Geometry: final body of the model. Coordinates: model frame, mm. Face numbers are marked on the shaded views. A direction names the side the tool comes from. Coordinates: 2 decimals unless noted, no trailing zeros. Loops run counter-clockwise (first coordinate to the right, second up) from the corner with the lowest first, then second, coordinate; pieces in that order, holes last. Notation, with made-up numbers: (61.25, 41.5) -> (80.25, 41.5) arc R19 cw to (80.25, 46.5) -> close; hole circle Ø10 at (7, -14). An arc over 180 degrees is marked (long way). One line per item, written item: value. Start each with the question number.
Item 1: Section query B-B on y = -4.5. Return loops of the section in (x, z).
Item 2: Mould query, pull axis Z, two halves, no side actions, for the marked faces 3, 4 and 5. Classes: +Z half, -Z half, draft (parallel to the pull), parting line (faces both ways), or undercut.
Item 3: Contact query for flat-ended pins moving along their axis: pin 1 Ø1.5 at (x, z) = (20, -10) entering from -Y; pin 2 Ø7.5 at (y, z) = (-12.7, 0) entering from -X; pin 3 Ø1 at (x, y) = (26.5, -13) entering from -Z. Output: stop coordinate, or through.
Item 4: Section query D-D on y = -12.7. Give the number of separate pieces and of enclosed holes in the cut face, then the cut area to 3 significant figures.
Item 5: Set-up query: the marked faces 1 and 2. Return all of +Z, -Z, +X, -X, +Y, -Y with unobstructed straight access to the full face (end or side cutting, diameter ignored); none if empty.
Item 6: Ray query, probe 1 along X at (y, z) = (-10.5, 7); probe 2 along Y at (x, z) = (0, 49) (3 decimals). Return the intervals inside material, ascending. Write a range as from..to.
Item 7: Section query C-C on z = 0. Return loops of the section in (x, y).
Item 8: Section query A-A on x = 0. Return loops of the section in (y, z) (3 decimals), then the cut area to 3 significant figures.
from build123d import *

# Parameters (mm, degrees)
F1_DEPTH = 25.4
F2_T     = -2.54
F4_D     = 6.35
F6_D     = 12.7


with BuildPart() as f1:
    # F0 (on Front) → F1 (new body)
    with BuildSketch(Plane.XZ):
        Polygon((50.8, -21.042049), (50.8, 21.042049), (21.042049, 50.8), (-21.042049, 50.8), (-21.042049, -50.8), (0, -50.8), (21.042049, -50.8), align=None)
        Polygon((-21.042049, -50.8), (-21.042049, 50.8), (-50.8, 21.042049), (-50.8, -21.042049), align=None)
    extrude(amount=F1_DEPTH)

    # F2
    f2_openings = [f1.faces().sort_by_distance(p)[0] for p in [
        (0, -25.4, 0),
    ]]
    offset(amount=F2_T, openings=f2_openings)

    # F4 (through all)
    with Locations(Plane(origin=(0, 0, -50.8), x_dir=(1, 0, 0), z_dir=(0, 0, -1))):
        with Locations((0, 12.7)):
            Hole(F4_D / 2)

    # F6 (through all)
    with Locations(Plane.YZ.offset(50.8)):
        with Locations((-12.7, 0)):
            Hole(F6_D / 2)


solid = f1.part
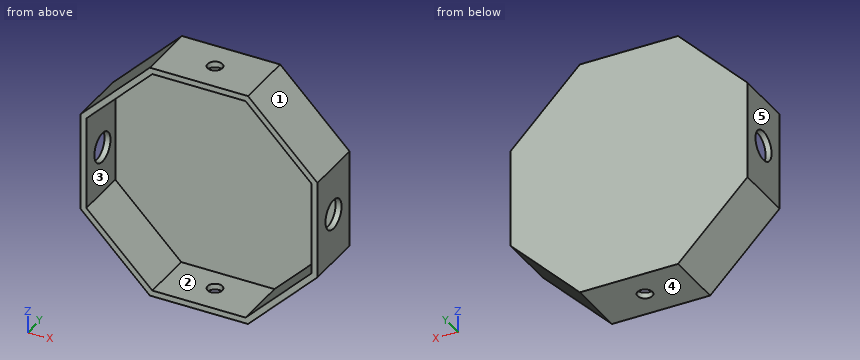
Reply:
1. outline: (-50.8, -21.04) -> (-21.04, -50.8) -> (21.04, -50.8) -> (50.8, -21.04) -> (50.8, 21.04) -> (21.04, 50.8) -> (-21.04, 50.8) -> (-50.8, 21.04) -> close; hole (-48.26, -19.99) -> (-19.99, -48.26) -> (19.99, -48.26) -> (48.26, -19.99) -> (48.26, 19.99) -> (19.99, 48.26) -> (-19.99, 48.26) -> (-48.26, 19.99) -> close
2. face 3: undercut
2. face 4: -Z half
2. face 5: draft
3. pin 1: stops at y = -2.54
3. pin 2: passes through
3. pin 3: stops at z = -45.84
4. separate pieces: 4
4. enclosed holes: 0
4. area: 737 mm²
5. face 1: +Z, +X, +Y, -Y
5. face 2: -Y
6. probe 1: x = -50.8..-48.26, 48.26..50.8
6. probe 2: y = -25.4..-15.875, -9.525..0
7. outline: (-50.8, -25.4) -> (-48.26, -25.4) -> (-48.26, -19.05) -> (-50.8, -19.05) -> close; (-50.8, -6.35) -> (-48.26, -6.35) -> (-48.26, -2.54) -> (48.26, -2.54) -> (48.26, -6.35) -> (50.8, -6.35) -> (50.8, 0) -> (-50.8, 0) -> close; (48.26, -25.4) -> (50.8, -25.4) -> (50.8, -19.05) -> (48.26, -19.05) -> close
8. outline: (-25.4, -50.8) -> (-15.875, -50.8) -> (-15.875, -48.26) -> (-25.4, -48.26) -> close; (-25.4, 48.26) -> (-15.875, 48.26) -> (-15.875, 50.8) -> (-25.4, 50.8) -> close; (-9.525, -50.8) -> (0, -50.8) -> (0, 50.8) -> (-9.525, 50.8) -> (-9.525, 48.26) -> (-2.54, 48.26) -> (-2.54, -48.26) -> (-9.525, -48.26) -> close
8. area: 342 mm²
